The drawing under review shows one solid part. Ordinate dimensions are in mm from its lowest x, y, z. Coordinates: 2 decimals unless noted, no trailing zeros. Write each loop counter-clockwise with the first axis right and the second up, starting at its lowest first coordinate (ties: lowest second). Pieces come first, ordered by that corner, then holes.
Q1. Take a section at A-A (z = 35). Give the boundary of the cut face in (x, y), and give its area (3 significant figures).
Q2. Take a section at B-B (y = 35). Give the boundary of the cut face in (x, z).
Q3. Take a section at D-D (y = 60.5). Give the boundary of the cut face in (x, z), and give its area (3 significant figures).
Q4. Insertion check: pin 1 (5 mm diameter, centred on x = 6.5, y = 22, fed in from +Z); pin 2 (2 mm diameter, centred on x = 9, y = 11.5, fed in from -Z); pin 3 (1.5 mm diameter, centred on x = 6, y = 22.5, fed in from -Z). Each pin has a flat end and moves straight along its axis. Give the tip position at first contact, or say it passes through.
Q5. For probe 1 along Y at (x, z) = (9, 36); probe 2 along Z at (x, y) = (9.5, 64); probe 3 along Z at (x, y) = (5.25, 45.5), list the stretches that pass through material, from the lowest coordinate up.
Q6. Take a section at C-C (x = 4). Give the boundary of the cut face in (y, z), and give its area (3 significant figures).
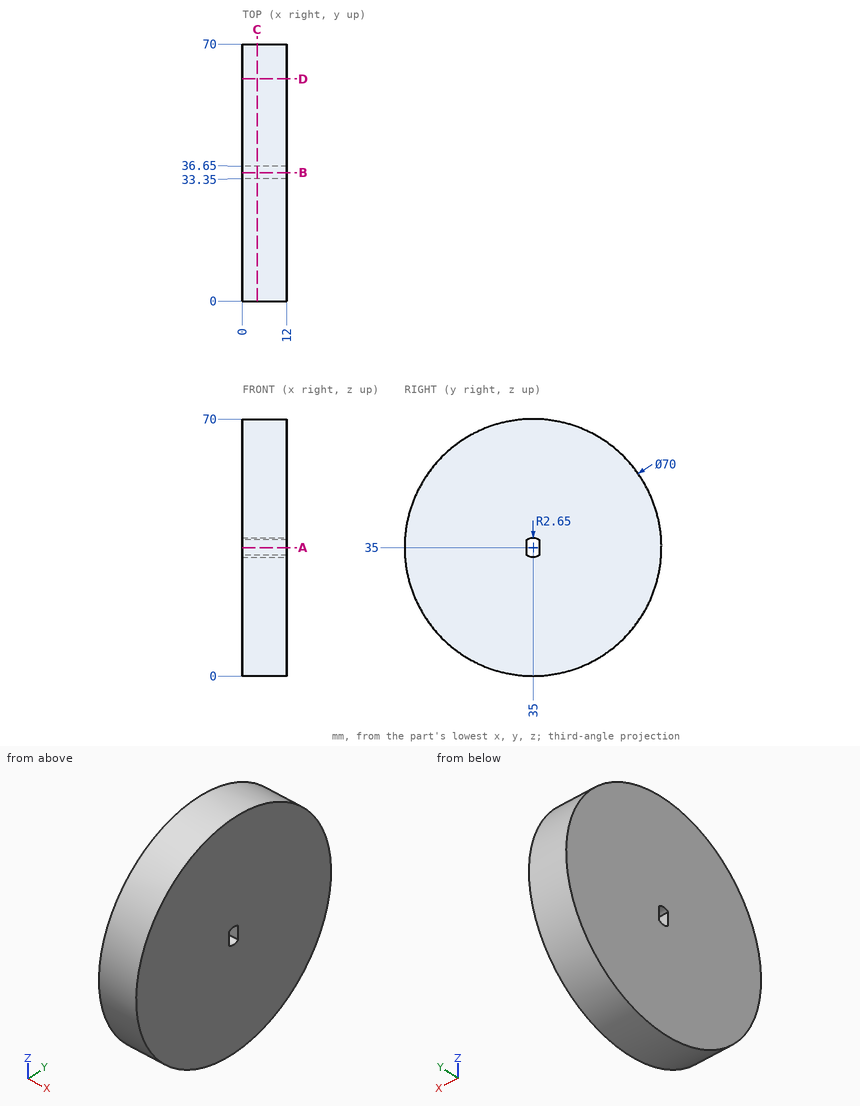
Response:
1. outline: (0, 0) - (12, 0) - (12, 33.35) - (0, 33.35) - close; (0, 36.65) - (12, 36.65) - (12, 70) - (0, 70) - close
1. area: 800 mm2
2. outline: (0, 0) - (12, 0) - (12, 32.35) - (0, 32.35) - close; (0, 37.65) - (12, 37.65) - (12, 70) - (0, 70) - close
3. outline: (0, 11.03) - (12, 11.03) - (12, 58.97) - (0, 58.97) - close
3. area: 575 mm2
4. pin 1: stops at z = 68.39
4. pin 2: stops at z = 8.19
4. pin 3: stops at z = 2.03
5. probe 1: y = 0.01 to 33.35, 36.65 to 69.99
5. probe 2: z = 15.4 to 54.6
5. probe 3: z = 1.61 to 68.39
6. outline: circle Ø70 at (35, 35); hole (33.35, 32.93) arc R2.65 ccw to (36.65, 32.93) - (36.65, 37.07) arc R2.65 ccw to (33.35, 37.07) - close
6. area: 3,830 mm2
